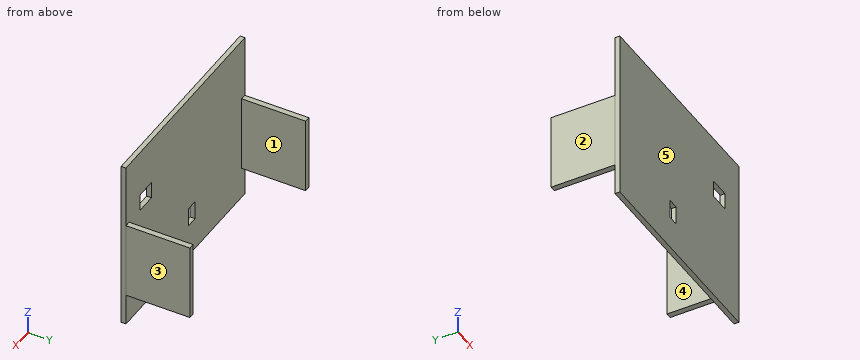
from build123d import *

# Parameters (mm, degrees)
SKETCH1_W           = 56
SKETCH1_H           = 46
BOSS_EXTRUDE1_DEPTH = 1.27
SKETCH2_W           = 1.5
SKETCH2_H           = 20.5
BOSS_EXTRUDE2_DEPTH = 17
SKETCH3_W           = 3
SKETCH3_H           = 5
CUT_EXTRUDE1_DEPTH  = 17
SKETCH4_W           = 5.5
SKETCH4_H           = 4.5
CUT_EXTRUDE2_DEPTH  = 17


with BuildPart() as part:
    # Sketch1 → Boss-Extrude1 (new body)
    with BuildSketch(Plane(origin=(0, 0, 0), x_dir=(1, 0, 0), z_dir=(0, 1, 0))):
        Rectangle(SKETCH1_W, SKETCH1_H)
    extrude(amount=BOSS_EXTRUDE1_DEPTH)

    # Sketch2 → Boss-Extrude2 (add)
    with BuildSketch(Plane(origin=(0, 1.27, 0), x_dir=(1, 0, 0), z_dir=(0, 1, 0))):
        with Locations((-27.248, 4.25)):
            Rectangle(SKETCH2_W, SKETCH2_H)
    boss_extrude2 = extrude(amount=BOSS_EXTRUDE2_DEPTH)

    # Mirror2: Boss-Extrude2 across plane
    add(boss_extrude2.mirror(Plane(origin=(0, 0, 0), x_dir=(0, 0, 1), z_dir=(1, 0, 0))))

    # Sketch3 → Cut-Extrude1 (cut)
    with BuildSketch(Plane(origin=(0, 1.27, 0), x_dir=(1, 0, 0), z_dir=(0, 1, 0))):
        with Locations((-2.998, 11.743007137)):
            Rectangle(SKETCH3_W, SKETCH3_H)
    extrude(amount=-CUT_EXTRUDE1_DEPTH, mode=Mode.SUBTRACT)

    # Sketch4 → Cut-Extrude2 (cut)
    with BuildSketch(Plane(origin=(0, 1.27, 0), x_dir=(1, 0, 0), z_dir=(0, 1, 0))):
        with Locations((18.748, -8.25)):
            Rectangle(SKETCH4_W, SKETCH4_H)
    extrude(amount=-CUT_EXTRUDE2_DEPTH, mode=Mode.SUBTRACT)


solid = part.part
Geometry: final body of the model. Coordinates: model frame, mm. Face numbers are marked on the shaded views. A direction names the side the tool comes from. Coordinates: 2 decimals unless noted, no trailing zeros. Order: outer loops, then holes, each group sorted by start corner. A loop starts at its lowest first (then second) coordinate and runs counter-clockwise, first axis right, second up.
(1) Access query for the marked faces 1 and 2. Directions: +Z, -Z, +X, -X, +Y, -Y. A direction counts if a zero-diameter tool reaches every point of the face in a straight line with its end or side. Return the directions, or none.
(2) Section query A-A (y = 12). Return the cut outline in (x, z).
(3) Material intervals for probe 1 along X at (y, z) = (6, -3); probe 2 along Y at (x, z) = (-21.5, 14), sorted ascending.
(4) First-contact query: pin 1 (3 mm diameter, centred on x = -1.5, z = 1.5, fed in from +Y); pin 2 (1.2 mm diameter, centred on x = 27.5, y = 5.5, fed in from -Z). Flat tips, straight axial feed; report the tip coordinate or a pass-through.
(5) Draft query along X for the marked faces 3, 4 and 5. Return one class per face: pulls with the +X half, pulls with the -X half, needs draft (parallel to the pull), parting line crosses it, or undercut.
(6) Section query D-D (x = -12). Return the cut outline in (y, z), plus the area to 3 significant figures.
Solution:
1. face 1: +Z, -Z, +Y
1. face 2: +Z, -Z, -X, +Y, -Y
2. outline: (-28, -14.5) - (-26.5, -14.5) - (-26.5, 6) - (-28, 6) - close; (26.5, -14.5) - (28, -14.5) - (28, 6) - (26.5, 6) - close
3. probe 1: x = -28 to -26.5, 26.5 to 28
3. probe 2: y = 0 to 1.27
4. pin 1: stops at y = 1.27
4. pin 2: stops at z = -14.5
5. face 3: pulls with the +X half
5. face 4: undercut
5. face 5: needs draft
6. outline: (0, -23) - (1.27, -23) - (1.27, 23) - (0, 23) - close
6. area: 58.4 mm2
